Read the model definition and answer for the solid it produces. Units are mm, in the model's axes. Give positions to 0.01 mm unless a question says otherwise; leave off trailing zeros. Write each loop counter-clockwise with the first axis right and the second up, starting at its lowest first coordinate (ties: lowest second). Pieces come first, ordered by that corner, then holes.
Autodesk Inventor part; units mm, degrees
ref_plane "YZ Plane" through (0, 0, 0) normal (1, 0, 0) x (0, 1, 0)
ref_plane "XZ Plane" through (0, 0, 0) normal (0, 1, 0) x (-1, 0, 0)
ref_plane "XY Plane" through (0, 0, 0) normal (0, 0, 1) x (1, 0, 0)
sketch "Sketch1" plane through (0, 0, 0) normal (1, 0, 0) x (0, 1, 0)
  line L0 (2, 0) -> (55.3, 0)
  line L1 (57.3, -2) -> (57.3, -55.3)
  line L2 (55.3, -57.3) -> (2, -57.3)
  line L3 (0, -55.3) -> (0, -2)
  arc A0 (57.3, -2) -> (55.3, 0) centre (55.3, -2) ccw
  arc A1 (55.3, -57.3) -> (57.3, -55.3) centre (55.3, -55.3) ccw
  arc A2 (0, -55.3) -> (2, -57.3) centre (2, -55.3) ccw
  arc A3 (2, 0) -> (0, -2) centre (2, -2) ccw
  line L4 (52.22, -5.08) -> (5.08, -5.08) construction
  line L5 (5.08, -5.08) -> (5.08, -52.22) construction
  line L6 (5.08, -52.22) -> (52.22, -52.22) construction
  line L7 (52.22, -52.22) -> (52.22, -5.08) construction
  line L8 (52.22, -5.08) -> (57.3, -5.08) construction
  line L9 (52.22, -5.08) -> (52.22, 0) construction
  line L10 (5.08, -52.22) -> (0, -52.22) construction
  line L11 (5.08, -52.22) -> (5.08, -57.3) construction
  circle A4 centre (52.22, -5.08) radius 2.5
  circle A5 centre (52.22, -52.22) radius 2.5
  circle A6 centre (5.08, -52.22) radius 2.5
  circle A7 centre (5.08, -5.08) radius 2.5
  point P0 (0, 0)
  point P1 (57.3, -57.3)
  point P2 (57.3, 0)
  point P3 (0, -57.3)
  dimension "d0" = 57.3
  dimension "d1" = 57.3
  dimension "d2" = 2
  dimension "d3" = 2
  dimension "d4" = 5
  dimension "d5" = 5
  dimension "d6" = 5
  dimension "d7" = 5
  dimension "d8" = 47.14
  dimension "d9" = 47.14
extrude "Extrusion1" add sketch "Sketch1" along normal blind 5.5
sketch "Sketch2" plane through (0, 0, 0) normal (-1, 0, 0) x (0, 0, 1)
  line L0 (-57.3, 2) -> (-57.3, 55.3) construction
  arc A0 (-57.3, 2) -> (-55.3, 0) centre (-55.3, 2) ccw
  line L1 (-2, 0) -> (-55.3, 0) construction
  arc A1 (-2, 0) -> (0, 2) centre (-2, 2) ccw
  line L2 (0, 55.3) -> (0, 2) construction
  arc A2 (0, 55.3) -> (-2, 57.3) centre (-2, 55.3) ccw
  line L3 (-55.3, 57.3) -> (-2, 57.3) construction
  arc A3 (-55.3, 57.3) -> (-57.3, 55.3) centre (-55.3, 55.3) ccw
  circle A4 centre (-5.08, 52.22) radius 2.5
  circle A5 centre (-52.22, 52.22) radius 2.5
  circle A6 centre (-52.22, 5.08) radius 2.5
  circle A7 centre (-5.08, 5.08) radius 2.5
  line L4 (-55.3, 57.3) -> (-2, 57.3) construction
  line L5 (-47.65, 57.3) -> (-9.65, 57.3)
  line L6 (-57.3, 2) -> (-57.3, 55.3) construction
  line L7 (-57.3, 9.65) -> (-57.3, 47.65)
  line L8 (-2, 0) -> (-55.3, 0) construction
  line L9 (-47.65, 0) -> (-9.65, 0)
  line L10 (0, 9.65) -> (0, 47.65)
  line L11 (0, 55.3) -> (0, 2) construction
  circle A8 centre (-52.22, 5.08) radius 2.5 construction
  line L12 (-52.22, 5.08) -> (-5.08, 52.22) construction
  line L13 (-28.65, 28.65) -> (-28.65, 57.3) construction
  line L14 (-28.65, 28.65) -> (-28.65, 0) construction
  line L15 (-28.65, 28.65) -> (0, 28.65) construction
  line L16 (-28.65, 28.65) -> (-57.3, 28.65) construction
  arc A9 (-51.5421, 47.65) -> (-47.6, 52.22) centre (-52.22, 52.22) ccw
  arc A10 (-9.7, 52.22) -> (-5.7579, 47.65) centre (-5.08, 52.22) ccw
  arc A11 (-5.7579, 9.65) -> (-9.7, 5.08) centre (-5.08, 5.08) ccw
  arc A12 (-47.6, 5.08) -> (-51.5421, 9.65) centre (-52.22, 5.08) ccw
  line L17 (-47.65, 57.3) -> (-47.6, 52.22)
  line L18 (-57.3, 47.65) -> (-51.5421, 47.65)
  line L19 (-9.7, 5.08) -> (-9.65, 0)
  line L20 (0, 9.65) -> (-5.7579, 9.65)
  line L21 (-9.6451, 47.6951) -> (-9.6048, 47.6952)
  line L22 (-5.7579, 47.65) -> (0, 47.65)
  line L23 (-9.65, 57.3) -> (-9.7, 52.22)
  line L24 (-9.6451, 47.6951) -> (-9.6451, 47.6549)
  line L25 (-47.6048, 9.6549) -> (-47.6452, 9.6548)
  line L26 (-51.5421, 9.65) -> (-57.3, 9.65)
  line L27 (-47.6049, 9.6951) -> (-47.6048, 9.6549)
  line L28 (-47.6, 5.08) -> (-47.65, 0)
  arc A13 (-56.05, 47.65) -> (-57.3, 46.4) centre (-56.05, 46.4) ccw
  arc A14 (-46.3876, 57.3) -> (-47.6376, 56.0377) centre (-46.3876, 56.05) ccw
  arc A15 (-9.6624, 56.0377) -> (-10.9124, 57.3) centre (-10.9124, 56.05) ccw
  arc A16 (0, 46.4) -> (-1.25, 47.65) centre (-1.25, 46.4) ccw
  arc A17 (-1.25, 9.65) -> (0, 10.9) centre (-1.25, 10.9) ccw
  arc A18 (-10.9124, 0) -> (-9.6624, 1.2623) centre (-10.9124, 1.25) ccw
  arc A19 (-47.6376, 1.2623) -> (-46.3876, 0) centre (-46.3876, 1.25) ccw
  arc A20 (-57.3, 10.9) -> (-56.05, 9.65) centre (-56.05, 10.9) ccw
  line L29 (-55.3, 57.3) -> (-2, 57.3)
  line L30 (-57.3, 2) -> (-57.3, 55.3)
  line L31 (0, 55.3) -> (0, 2)
  point P0 (0, 0)
  point P1 (-10.9124, 57.3)
  dimension "d12" = 38
  dimension "d13" = 38
  dimension "d14" = 38
  dimension "d15" = 38
  dimension "d16" = 2.12
  dimension "d17" = 2.12
  dimension "d18" = 2.12
  dimension "d19" = 2.12
  dimension "d20" = 2.5
  dimension "d21" = 2.5
  dimension "d22" = 2.5
  dimension "d23" = 2.5
  dimension "d24" = 2.5
  dimension "d25" = 2.5
  dimension "d26" = 2.5
  dimension "d27" = 2.5
extrude "Extrusion2" add sketch "Sketch2" along normal blind 5.5 contours L10 A17 L20 A11 L19 A18 L9 A19 L28 A12 L26 A20 L7 A13 L18 A9 L17 A14 L5 A15 L23 A10 L22 A16
sketch "Sketch3" plane through (-5.5, 0, 0) normal (-1, 0, 0) x (0, 0, 1)
  line L0 (-51.5421, 47.65) -> (-56.05, 47.65)
  arc A0 (-56.05, 47.65) -> (-57.3, 46.4) centre (-56.05, 46.4) ccw
  line L1 (-57.3, 46.4) -> (-57.3, 10.9)
  arc A1 (-57.3, 10.9) -> (-56.05, 9.65) centre (-56.05, 10.9) ccw
  line L2 (-56.05, 9.65) -> (-51.5421, 9.65)
  arc A2 (-47.6, 5.08) -> (-51.5421, 9.65) centre (-52.22, 5.08) ccw
  line L3 (-47.6, 5.08) -> (-47.6376, 1.2623)
  arc A3 (-47.6376, 1.2623) -> (-46.3876, 0) centre (-46.3876, 1.25) ccw
  line L4 (-46.3876, 0) -> (-10.9124, 0)
  arc A4 (-10.9124, 0) -> (-9.6624, 1.2623) centre (-10.9124, 1.25) ccw
  line L5 (-9.6624, 1.2623) -> (-9.7, 5.08)
  arc A5 (-5.7579, 9.65) -> (-9.7, 5.08) centre (-5.08, 5.08) ccw
  line L6 (-5.7579, 9.65) -> (-1.25, 9.65)
  arc A6 (-1.25, 9.65) -> (0, 10.9) centre (-1.25, 10.9) ccw
  line L7 (0, 10.9) -> (0, 46.4)
  arc A7 (0, 46.4) -> (-1.25, 47.65) centre (-1.25, 46.4) ccw
  line L8 (-1.25, 47.65) -> (-5.7579, 47.65)
  arc A8 (-9.7, 52.22) -> (-5.7579, 47.65) centre (-5.08, 52.22) ccw
  line L9 (-9.7, 52.22) -> (-9.6624, 56.0377)
  arc A9 (-9.6624, 56.0377) -> (-10.9124, 57.3) centre (-10.9124, 56.05) ccw
  line L10 (-10.9124, 57.3) -> (-46.3876, 57.3)
  arc A10 (-46.3876, 57.3) -> (-47.6376, 56.0377) centre (-46.3876, 56.05) ccw
  line L11 (-47.6376, 56.0377) -> (-47.6, 52.22)
  arc A11 (-51.5421, 47.65) -> (-47.6, 52.22) centre (-52.22, 52.22) ccw
  line L12 (-46.3876, 57.2) -> (-10.9124, 57.2)
  arc A12 (-9.7624, 56.0387) -> (-10.9124, 57.2) centre (-10.9124, 56.05) ccw
  line L13 (-9.7624, 56.0387) -> (-9.8, 52.2205)
  arc A13 (-9.8, 52.2205) -> (-5.7652, 47.55) centre (-5.08, 52.22) ccw
  line L14 (-5.7652, 47.55) -> (-1.25, 47.55)
  arc A14 (-0.1, 46.4) -> (-1.25, 47.55) centre (-1.25, 46.4) ccw
  line L15 (-0.1, 46.4) -> (-0.1, 10.9)
  arc A15 (-1.25, 9.75) -> (-0.1, 10.9) centre (-1.25, 10.9) ccw
  line L16 (-1.25, 9.75) -> (-5.7652, 9.75)
  arc A16 (-5.7652, 9.75) -> (-9.8, 5.0795) centre (-5.08, 5.08) ccw
  line L17 (-9.8, 5.0795) -> (-9.7624, 1.2613)
  arc A17 (-10.9124, 0.1) -> (-9.7624, 1.2613) centre (-10.9124, 1.25) ccw
  line L18 (-10.9124, 0.1) -> (-46.3876, 0.1)
  arc A18 (-47.5376, 1.2613) -> (-46.3876, 0.1) centre (-46.3876, 1.25) ccw
  line L19 (-47.5376, 1.2613) -> (-47.5, 5.0795)
  arc A19 (-47.5, 5.0795) -> (-51.5348, 9.75) centre (-52.22, 5.08) ccw
  line L20 (-51.5348, 9.75) -> (-56.05, 9.75)
  arc A20 (-57.2, 10.9) -> (-56.05, 9.75) centre (-56.05, 10.9) ccw
  line L21 (-57.2, 10.9) -> (-57.2, 46.4)
  arc A21 (-56.05, 47.55) -> (-57.2, 46.4) centre (-56.05, 46.4) ccw
  line L22 (-56.05, 47.55) -> (-51.5348, 47.55)
  arc A22 (-51.5348, 47.55) -> (-47.5, 52.2205) centre (-52.22, 52.22) ccw
  line L23 (-47.5, 52.2205) -> (-47.5376, 56.0387)
  arc A23 (-46.3876, 57.2) -> (-47.5376, 56.0387) centre (-46.3876, 56.05) ccw
  point P0 (0, 0)
  dimension "d30" = 0.1
extrude "Extrusion3" add sketch "Sketch3" along normal blind 54.5 contours L12 A12 L13 A13 L14 A14 L15 A15 L16 A16 L17 A17 L18 A18 L19 A19 L20 A20 L21 A21 L22 A22 L23 A23
sketch "Sketch4" plane through (-60, 0, 0) normal (-1, 0, 0) x (0, 0, 1)
  arc A0 (-56.05, 47.55) -> (-57.2, 46.4) centre (-56.05, 46.4) ccw
  line L0 (-56.05, 47.55) -> (-51.5348, 47.55)
  arc A1 (-51.5348, 47.55) -> (-47.5, 52.2205) centre (-52.22, 52.22) ccw
  line L1 (-47.5, 52.2205) -> (-47.5376, 56.0387)
  arc A2 (-46.3876, 57.2) -> (-47.5376, 56.0387) centre (-46.3876, 56.05) ccw
  line L2 (-46.3876, 57.2) -> (-10.9124, 57.2)
  arc A3 (-9.7624, 56.0387) -> (-10.9124, 57.2) centre (-10.9124, 56.05) ccw
  line L3 (-9.7624, 56.0387) -> (-9.8, 52.2205)
  arc A4 (-9.8, 52.2205) -> (-5.7652, 47.55) centre (-5.08, 52.22) ccw
  line L4 (-5.7652, 47.55) -> (-1.25, 47.55)
  arc A5 (-0.1, 46.4) -> (-1.25, 47.55) centre (-1.25, 46.4) ccw
  line L5 (-0.1, 46.4) -> (-0.1, 10.9)
  arc A6 (-1.25, 9.75) -> (-0.1, 10.9) centre (-1.25, 10.9) ccw
  line L6 (-1.25, 9.75) -> (-5.7652, 9.75)
  arc A7 (-5.7652, 9.75) -> (-9.8, 5.0795) centre (-5.08, 5.08) ccw
  line L7 (-9.8, 5.0795) -> (-9.7624, 1.2613)
  arc A8 (-10.9124, 0.1) -> (-9.7624, 1.2613) centre (-10.9124, 1.25) ccw
  line L8 (-10.9124, 0.1) -> (-46.3876, 0.1)
  arc A9 (-47.5376, 1.2613) -> (-46.3876, 0.1) centre (-46.3876, 1.25) ccw
  line L9 (-47.5376, 1.2613) -> (-47.5, 5.0795)
  arc A10 (-47.5, 5.0795) -> (-51.5348, 9.75) centre (-52.22, 5.08) ccw
  line L10 (-51.5348, 9.75) -> (-56.05, 9.75)
  arc A11 (-57.2, 10.9) -> (-56.05, 9.75) centre (-56.05, 10.9) ccw
  line L11 (-57.2, 10.9) -> (-57.2, 46.4)
  line L12 (-51.5421, 47.65) -> (-56.05, 47.65)
  arc A12 (-56.05, 47.65) -> (-57.3, 46.4) centre (-56.05, 46.4) ccw
  line L13 (-57.3, 46.4) -> (-57.3, 10.9)
  arc A13 (-57.3, 10.9) -> (-56.05, 9.65) centre (-56.05, 10.9) ccw
  line L14 (-56.05, 9.65) -> (-51.5421, 9.65)
  arc A14 (-47.6, 5.08) -> (-51.5421, 9.65) centre (-52.22, 5.08) ccw
  line L15 (-47.6, 5.08) -> (-47.6376, 1.2623)
  arc A15 (-47.6376, 1.2623) -> (-46.3876, 0) centre (-46.3876, 1.25) ccw
  line L16 (-46.3876, 0) -> (-10.9124, 0)
  arc A16 (-10.9124, 0) -> (-9.6624, 1.2623) centre (-10.9124, 1.25) ccw
  line L17 (-9.6624, 1.2623) -> (-9.7, 5.08)
  arc A17 (-5.7579, 9.65) -> (-9.7, 5.08) centre (-5.08, 5.08) ccw
  line L18 (-5.7579, 9.65) -> (-1.25, 9.65)
  arc A18 (-1.25, 9.65) -> (0, 10.9) centre (-1.25, 10.9) ccw
  line L19 (0, 10.9) -> (0, 46.4)
  arc A19 (0, 46.4) -> (-1.25, 47.65) centre (-1.25, 46.4) ccw
  line L20 (-1.25, 47.65) -> (-5.7579, 47.65)
  arc A20 (-9.7, 52.22) -> (-5.7579, 47.65) centre (-5.08, 52.22) ccw
  line L21 (-9.7, 52.22) -> (-9.6624, 56.0377)
  arc A21 (-9.6624, 56.0377) -> (-10.9124, 57.3) centre (-10.9124, 56.05) ccw
  line L22 (-10.9124, 57.3) -> (-46.3876, 57.3)
  arc A22 (-46.3876, 57.3) -> (-47.6376, 56.0377) centre (-46.3876, 56.05) ccw
  line L23 (-47.6376, 56.0377) -> (-47.6, 52.22)
  arc A23 (-51.5421, 47.65) -> (-47.6, 52.22) centre (-52.22, 52.22) ccw
  point P0 (0, 0)
extrude "Extrusion4" add sketch "Sketch4" along normal blind 11 contours L0 A1 L1 A2 L2 A3 L3 A4 L4 A5 L5 A6 L6 A7 L7 A8 L8 A9 L9 A10 L10 A11 L11 A0 | A23 L23 A22 L22 A21 L21 A20 L20 A19 L19 A18 L18 A17 L17 A16 L16 A15 L15 A14 L14 A13 L13 A12 L12
sketch "Sketch5" plane through (5.5, 0, 0) normal (1, 0, 0) x (0, 0, -1)
  line L0 (46.3876, 57.2) -> (10.9124, 57.2) construction
  line L1 (28.65, 57.2) -> (28.65, 0.1) construction
  line L2 (10.9124, 0.1) -> (46.3876, 0.1) construction
  circle A0 centre (28.65, 28.65) radius 19.05
  point P0 (0, 0)
  dimension "d35" = 38.1
extrude "Extrusion5" add sketch "Sketch5" along normal blind 1.6
sketch "Sketch6" plane through (7.1, 28.65, -28.65) normal (1, 0, 0) x (0, 0, -1)
  circle A0 centre (0, 0) radius 3.175
  point P0 (-28.65, -28.65)
  dimension "d38" = 6.35
extrude "Extrusion6" add sketch "Sketch6" along normal blind 4.4
sketch "Sketch7" plane through (11.5, 28.65, -28.65) normal (1, 0, 0) x (0, 0, -1)
  circle A0 centre (0, 0) radius 3.175
  line L0 (-9.5378, 2.375) -> (9.1058, 2.375)
  point P0 (-28.65, -28.65)
  point P1 (2.1071, 2.375)
  point P2 (-2.1071, 2.375)
  dimension "d41" = 2.375
extrude "Extrusion7" add sketch "Sketch7" along normal blind 15 contours A0 L0 picked at (0.5748, 0.6947)
sketch "Sketch8" plane through (-60, 57.3, -10.9124) normal (0, 1, 0) x (1, 0, 0)
  line L0 (-11, 35.4753) -> (-11, 0)
  line L1 (0, 0) -> (0, 35.4753)
  line L2 (-11, 11.75) -> (0, 11.75)
  line L3 (0, 11.75) -> (0, 23.75)
  line L4 (0, 23.75) -> (-11, 23.75)
  line L5 (-11, 23.75) -> (-11, 11.75)
  point P0 (60, -10.9124)
  point P1 (-11, 23.75)
  point P2 (0, 11.75)
  dimension "d44" = 12
  dimension "d45" = 11.75
extrude "Extrusion8" add sketch "Sketch8" along normal blind 1.5
equation "\"d5\" = d4"
equation "\"d6\" = d4"
equation "\"d7\" = d4"
equation "\"d13\" = d12"
equation "\"d14\" = d12"
equation "\"d15\" = d12"
equation "\"d17\" = d16"
equation "\"d18\" = d16"
equation "\"d19\" = d16"
equation "\"d21\" = d20"
equation "\"d22\" = d20"
equation "\"d23\" = d20"
equation "\"d24\" = d20"
equation "\"d25\" = d20"
equation "\"d26\" = d20"
equation "\"d27\" = d20"
properties part number "Nema 23 76.5mm Stepper Motor"
Item 1: Each of these flat-tipped pins is pushed along its axis until it touches: pin 1 Ø8 at (x, z) = (-32.5, -29) entering from -Y; pin 2 Ø1 at (x, y) = (-40, 49.5) entering from -Z; pin 3 Ø5 at (x, z) = (-64.5, -4) entering from -Y. Where does it stop, or does it pass through?
Result set:
pin 1: stops at y = 0.1
pin 2: stops at z = -48.77
pin 3: stops at y = 9.48
Item 2: Section C-C (z = -28.65) is taken. Write down the section's boundary in (x, y) (3 decimals).
Result set:
outline: (-71, 0) - (-60, 0) - (-60, 0.1) - (-5.5, 0.1) - (-5.5, 0) - (5.5, 0) - (5.5, 9.6) - (7.1, 9.6) - (7.1, 25.475) - (26.5, 25.475) - (26.5, 31.025) - (11.5, 31.025) - (11.5, 31.825) - (7.1, 31.825) - (7.1, 47.7) - (5.5, 47.7) - (5.5, 57.3) - (-5.5, 57.3) - (-5.5, 57.2) - (-60, 57.2) - (-60, 58.8) - (-71, 58.8) - close
Item 3: Find the intervals of material crossed by line 1 along Z through (x, y) = (1.9, 52.22); line 2 along Y through (x, z) = (3, -5); line 3 along X through (y, z) = (3, -24), in increasing order.
Result set:
line 1: z = -57.3 to -54.72, -49.72 to -7.58, -2.58 to 0
line 2: y = 0 to 2.58, 7.58 to 49.72, 54.72 to 57.3
line 3: x = -71 to 5.5
Item 4: Section B-B (y = 28.65) is taken. Write down the section's boundary in (x, z) (3 decimals), and give its area (3 significant figures).
Result set:
outline: (-71, -57.3) - (-60, -57.3) - (-60, -57.2) - (-5.5, -57.2) - (-5.5, -57.3) - (5.5, -57.3) - (5.5, -47.7) - (7.1, -47.7) - (7.1, -31.825) - (26.5, -31.825) - (26.5, -25.475) - (7.1, -25.475) - (7.1, -9.6) - (5.5, -9.6) - (5.5, 0) - (-5.5, 0) - (-5.5, -0.1) - (-60, -0.1) - (-60, 0) - (-71, 0) - close
area: 4,560 mm2
Item 5: Section A-A (x = 2) is taken. Write down the section's boundary in (y, z).
Result set:
outline: (0, -55.3) arc R2 ccw to (2, -57.3) - (55.3, -57.3) arc R2 ccw to (57.3, -55.3) - (57.3, -2) arc R2 ccw to (55.3, 0) - (2, 0) arc R2 ccw to (0, -2) - close; hole circle Ø5 at (5.08, -52.22); hole circle Ø5 at (5.08, -5.08); hole circle Ø5 at (52.22, -52.22); hole circle Ø5 at (52.22, -5.08)
Item 6: Section D-D (x = -31.5) is taken. Write down the section's boundary in (y, z), and give its area (3 significant figures).
Result set:
outline: (0.1, -46.39) arc R1.15 ccw to (1.26, -47.54) - (5.08, -47.5) arc R4.72 cw to (9.75, -51.53) - (9.75, -56.05) arc R1.15 ccw to (10.9, -57.2) - (46.4, -57.2) arc R1.15 ccw to (47.55, -56.05) - (47.55, -51.53) arc R4.72 cw to (52.22, -47.5) - (56.04, -47.54) arc R1.15 ccw to (57.2, -46.39) - (57.2, -10.91) arc R1.15 ccw to (56.04, -9.76) - (52.22, -9.8) arc R4.72 cw to (47.55, -5.77) - (47.55, -1.25) arc R1.15 ccw to (46.4, -0.1) - (10.9, -0.1) arc R1.15 ccw to (9.75, -1.25) - (9.75, -5.77) arc R4.72 cw to (5.08, -9.8) - (1.26, -9.76) arc R1.15 ccw to (0.1, -10.91) - close
area: 2,900 mm2
Item 7: Determine the mould class of faces 1 (the cylindrical face through (-32.37, 8.2, -48.68)), 2 (the flat face through (5.5, 28, -9)), 3 (the flat face through (-32, 9.75, -54)), 4 (the flat face through (-65, 9.65, -54)) for opening direction X: pulls with the +X half, pulls with the -X half, needs draft (parallel to the pull), parting line crosses it, or undercut.
Result set:
face 1: undercut
face 2: pulls with the +X half
face 3: undercut
face 4: needs draft
